Here's how the part is built. I have some questions about the finished solid (model axes, mm). Give positions to 0.01 mm unless a question says otherwise; leave off trailing zeros. Write each loop counter-clockwise with the first axis right and the second up, starting at its lowest first coordinate (ties: lowest second). Pieces come first, ordered by that corner, then holes. Notation, with made-up numbers: M -13.75,-3 L -6.75,-3 A21 cw -6.75,20 Z; hole C 36,79 d10. An arc over 180 degrees is marked long. Use one line per item in the form item = value. Start each with the question number.
Autodesk Inventor part; units mm, degrees
ref_plane "YZ Plane" through (0, 0, 0) normal (1, 0, 0) x (0, 1, 0)
ref_plane "XZ Plane" through (0, 0, 0) normal (0, 1, 0) x (-1, 0, 0)
ref_plane "XY Plane" through (0, 0, 0) normal (0, 0, 1) x (1, 0, 0)
sketch "Sketch1" plane through (0, 0, 0) normal (0, 1, 0) x (-1, 0, 0)
  point P0 (0, 0)
sketch "Sketch4" plane through (0, 0, 0) normal (0, 1, 0) x (-1, 0, 0)
  line L0 (-203.2, 0) -> (-203.2, -254)
  line L1 (-203.2, -254) -> (0, -254)
  line L2 (0, -254) -> (0, 0)
  line L3 (-101.6, 44.45) -> (-50.8, 44.45)
  line L4 (-50.8, 44.45) -> (0, 0)
  line L5 (-101.6, 44.45) -> (-152.4, 44.45)
  line L6 (-152.4, 44.45) -> (-203.2, 0)
  line L7 (-152.4, 44.45) -> (-136.0714, 58.7375)
  line L8 (-50.8, 44.45) -> (-67.1286, 58.7375)
  line L9 (-67.1286, 58.7375) -> (-136.0714, 58.7375)
  line L10 (0, -254) -> (0, -241.3)
  line L11 (-3.175, -241.3) -> (-3.175, -222.25)
  line L12 (-3.175, -222.25) -> (-9.525, -222.25)
  line L13 (-9.525, -222.25) -> (-9.525, -241.3)
  line L14 (-9.525, -241.3) -> (-3.175, -241.3)
  circle A0 centre (-6.35, -215.9) radius 4.7625
  circle A1 centre (-6.35, -215.9) radius 1.9844
  line L15 (-6.35, -209.55) -> (-9.525, -209.55)
  line L16 (-6.35, -209.55) -> (-3.175, -209.55)
  line L17 (-3.175, -209.55) -> (-3.175, -190.5)
  line L18 (-3.175, -190.5) -> (-9.525, -190.5)
  line L19 (-9.525, -190.5) -> (-9.525, -209.55)
  line L20 (-200.025, -241.3) -> (-200.025, -222.25)
  line L21 (-200.025, -222.25) -> (-193.675, -222.25)
  line L22 (-193.675, -222.25) -> (-193.675, -241.3)
  line L23 (-193.675, -241.3) -> (-200.025, -241.3)
  circle A2 centre (-196.85, -215.9) radius 4.7625
  circle A3 centre (-196.85, -215.9) radius 1.9844
  line L24 (-196.85, -209.55) -> (-193.675, -209.55)
  line L25 (-196.85, -209.55) -> (-200.025, -209.55)
  line L26 (-200.025, -209.55) -> (-200.025, -190.5)
  line L27 (-200.025, -190.5) -> (-193.675, -190.5)
  line L28 (-193.675, -190.5) -> (-193.675, -209.55)
  line L29 (-3.175, -63.5) -> (-3.175, -82.55)
  line L30 (-3.175, -82.55) -> (-9.525, -82.55)
  line L31 (-9.525, -82.55) -> (-9.525, -63.5)
  line L32 (-9.525, -63.5) -> (-3.175, -63.5)
  circle A4 centre (-6.35, -88.9) radius 4.7625
  circle A5 centre (-6.35, -88.9) radius 1.9844
  line L33 (-6.35, -95.25) -> (-9.525, -95.25)
  line L34 (-6.35, -95.25) -> (-3.175, -95.25)
  line L35 (-3.175, -95.25) -> (-3.175, -114.3)
  line L36 (-3.175, -114.3) -> (-9.525, -114.3)
  line L37 (-9.525, -114.3) -> (-9.525, -95.25)
  line L38 (-193.675, -63.5) -> (-200.025, -63.5)
  line L39 (-200.025, -63.5) -> (-200.025, -82.55)
  line L40 (-193.675, -82.55) -> (-193.675, -63.5)
  line L41 (-200.025, -82.55) -> (-193.675, -82.55)
  circle A6 centre (-196.85, -88.9) radius 4.7625
  line L42 (-196.85, -95.25) -> (-200.025, -95.25)
  line L43 (-196.85, -95.25) -> (-193.675, -95.25)
  line L44 (-200.025, -95.25) -> (-200.025, -114.3)
  line L45 (-200.025, -114.3) -> (-193.675, -114.3)
  line L46 (-193.675, -114.3) -> (-193.675, -95.25)
  circle A7 centre (-196.85, -88.9) radius 1.9844
  dimension "d18" = 203.2
  dimension "d19" = 254
  dimension "d29" = 19.05
  dimension "d30" = 6.35
  dimension "d32" = 9.525
  dimension "d33" = 3.9688
  dimension "d35" = 3.175
  dimension "d36" = 19.05
extrude "Extrusion2" add sketch "Sketch4" along normal blind 5.5563 contours L6 L5 L3 L4 L2 L1 L0 | L7 L9 L8 L3 L5 | A0 | A2 | A4 | A6
sketch "Sketch5" plane through (0, 5.5563, 0) normal (0, 1, 0) x (1, 0, 0)
  line L0 (67.1286, -58.7375) -> (136.0714, -58.7375)
  line L1 (136.0714, -58.7375) -> (129.7214, -58.7375)
  line L2 (129.7214, -58.7375) -> (129.7214, -52.3875)
  line L3 (129.7214, -52.3875) -> (117.0214, -52.3875)
  line L4 (117.0214, -52.3875) -> (117.0214, -58.7375)
  line L5 (117.0214, -58.7375) -> (104.3214, -58.7375)
  line L6 (0, 0) -> (67.1286, -58.7375)
  line L7 (67.1286, -58.7375) -> (73.4786, -58.7375)
  line L8 (73.4786, -58.7375) -> (73.4786, -52.3875)
  line L9 (73.4786, -52.3875) -> (86.1786, -52.3875)
  line L10 (86.1786, -52.3875) -> (86.1786, -58.7375)
  line L11 (86.1786, -58.7375) -> (101.5964, -58.7375)
  line L12 (101.5964, -52.3875) -> (95.2464, -52.3875)
  line L13 (101.5964, -52.3875) -> (107.9464, -52.3875)
  line L14 (107.9464, -52.3875) -> (107.9464, -58.7375)
  line L15 (95.2464, -52.3875) -> (95.2464, -58.7375)
  line L16 (73.4786, -58.7375) -> (86.1786, -58.7375)
extrude "Extrusion3" cut sketch "Sketch5" against normal blind 25.4
sketch "Sketch6" plane through (0, 5.5563, 0) normal (0, 1, 0) x (1, 0, 0)
  line L0 (73.4786, -52.3875) -> (86.1786, -52.3875)
  line L1 (73.4786, -46.0375) -> (73.4786, -39.6875)
  line L2 (73.4786, -39.6875) -> (73.4786, -46.0375)
  line L3 (129.74, -46.0375) -> (129.74, -39.6875)
  line L4 (129.74, -39.6875) -> (129.74, -46.0375)
  line L5 (86.1786, -46.0375) -> (86.1786, -39.6875)
  line L6 (95.2464, -46.0375) -> (95.2464, -39.6875)
  line L7 (117.0167, -46.0375) -> (117.0167, -39.6875)
  line L8 (107.95, -46.0375) -> (107.95, -39.6875)
  line L9 (73.4786, -39.6875) -> (86.1786, -39.6875)
  line L10 (95.2464, -39.6875) -> (107.95, -39.6875)
  line L11 (117.0167, -39.6875) -> (129.74, -39.6875)
  line L12 (129.74, -46.0375) -> (117.0167, -46.0375)
  line L13 (107.95, -46.0375) -> (95.2464, -46.0375)
  line L14 (86.1786, -46.0375) -> (73.4786, -46.0375)
  point P0 (0, 0)
  point P1 (95.2464, -52.3875)
extrude "Extrusion4" cut sketch "Sketch6" against normal blind 25.4
sketch "Sketch7" plane through (0, 5.5563, 0) normal (0, 1, 0) x (1, 0, 0)
  line L0 (3.175, 63.5) -> (3.175, 82.55)
  line L1 (3.175, 73.025) -> (8.7313, 73.025)
  line L2 (9.525, 82.55) -> (3.175, 82.55)
  line L3 (3.175, 63.5) -> (9.525, 63.5)
  line L4 (9.525, 82.55) -> (8.7313, 82.55)
  line L5 (8.7313, 82.55) -> (8.7313, 63.5)
  line L6 (8.7313, 63.5) -> (9.525, 63.5)
  line L7 (9.525, 63.5) -> (9.525, 82.55)
  line L8 (9.525, 114.3) -> (8.7313, 114.3)
  line L9 (8.7313, 114.3) -> (8.7313, 95.25)
  line L10 (8.7313, 95.25) -> (9.525, 95.25)
  line L11 (9.525, 95.25) -> (9.525, 114.3)
  line L12 (3.175, 209.55) -> (9.525, 209.55)
  line L13 (3.175, 190.5) -> (9.525, 190.5)
  line L14 (9.525, 209.55) -> (8.7313, 209.55)
  line L15 (8.7313, 209.55) -> (8.7313, 190.5)
  line L16 (8.7313, 190.5) -> (9.525, 190.5)
  line L17 (9.525, 190.5) -> (9.525, 209.55)
  line L18 (9.525, 241.3) -> (9.525, 222.25)
  line L19 (9.525, 241.3) -> (9.1281, 241.3)
  line L20 (9.1281, 222.25) -> (9.525, 222.25)
  line L21 (9.525, 222.25) -> (9.525, 241.3)
  line L22 (3.175, 222.25) -> (3.175, 241.3)
  line L23 (9.525, 241.3) -> (8.7313, 241.3)
  line L24 (8.7313, 241.3) -> (8.7313, 222.25)
  line L25 (8.7313, 222.25) -> (9.525, 222.25)
  line L26 (9.525, 222.25) -> (9.525, 241.3)
  line L27 (200.025, 241.3) -> (200.025, 222.25)
  line L28 (200.025, 231.775) -> (194.4688, 231.775)
  line L29 (193.675, 241.3) -> (193.675, 222.25)
  line L30 (193.675, 241.3) -> (194.4688, 241.3)
  line L31 (194.4688, 241.3) -> (194.4688, 222.25)
  line L32 (194.4688, 222.25) -> (193.675, 222.25)
  line L33 (193.675, 222.25) -> (193.675, 241.3)
  line L34 (193.675, 209.55) -> (193.675, 190.5)
  line L35 (200.025, 190.5) -> (193.675, 190.5)
  line L36 (193.675, 209.55) -> (194.4688, 209.55)
  line L37 (194.4688, 209.55) -> (194.4688, 190.5)
  line L38 (194.4688, 190.5) -> (193.675, 190.5)
  line L39 (193.675, 190.5) -> (193.675, 209.55)
  line L40 (193.675, 114.3) -> (194.4688, 114.3)
  line L41 (194.4688, 114.3) -> (194.4688, 95.25)
  line L42 (194.4688, 95.25) -> (193.675, 95.25)
  line L43 (193.675, 95.25) -> (193.675, 114.3)
  line L44 (193.675, 82.55) -> (193.675, 63.5)
  line L45 (193.675, 82.55) -> (194.4688, 82.55)
  line L46 (194.4688, 82.55) -> (194.4688, 63.5)
  line L47 (194.4688, 63.5) -> (193.675, 63.5)
  line L48 (193.675, 63.5) -> (193.675, 82.55)
  line L49 (86.1786, -52.3875) -> (86.1786, -58.7375)
  line L50 (73.4786, -52.3875) -> (73.4786, -58.7375)
  line L51 (86.1786, -52.3875) -> (73.4786, -52.3875)
  line L52 (73.4786, -52.3875) -> (73.4786, -53.1813)
  line L53 (73.4786, -53.1813) -> (86.1786, -53.1813)
  line L54 (86.1786, -53.1813) -> (86.1786, -52.3875)
  line L55 (95.2464, -58.7375) -> (95.2464, -52.3875)
  line L56 (107.9464, -52.3875) -> (107.9464, -58.7375)
  line L57 (95.2464, -52.3875) -> (107.9464, -52.3875)
  line L58 (107.9464, -52.3875) -> (107.9464, -53.1813)
  line L59 (107.9464, -53.1813) -> (95.2464, -53.1813)
  line L60 (95.2464, -53.1813) -> (95.2464, -52.3875)
  line L61 (117.0214, -52.3875) -> (130.175, -52.3875)
  line L62 (130.175, -52.3875) -> (130.175, -53.1813)
  line L63 (130.175, -53.1813) -> (117.0214, -53.1813)
  line L64 (117.0214, -53.1813) -> (117.0214, -52.3875)
  line L65 (86.1786, -46.0375) -> (86.1786, -39.6875)
  line L66 (73.4786, -39.6875) -> (86.1786, -39.6875)
  line L67 (86.1786, -39.6875) -> (86.1786, -40.4853)
  line L68 (86.1786, -40.4853) -> (73.4786, -40.4853)
  line L69 (73.4786, -40.4853) -> (73.4786, -39.6875)
  line L70 (95.2464, -39.6875) -> (107.9464, -39.6875)
  line L71 (107.9464, -39.6875) -> (107.9464, -40.4853)
  line L72 (107.9464, -40.4853) -> (95.2464, -40.4853)
  line L73 (95.2464, -40.4853) -> (95.2464, -39.6875)
  line L74 (117.0214, -39.6875) -> (129.74, -39.6875)
  line L75 (129.74, -39.6875) -> (129.74, -40.4853)
  line L76 (129.74, -40.4853) -> (117.0214, -40.4853)
  line L77 (117.0214, -40.4853) -> (117.0214, -39.6875)
  point P0 (0, 0)
  dimension "d65" = 5.5563
  dimension "d67" = 5.5563
extrude "Extrusion5" add sketch "Sketch7" against normal blind 5.5563 contours L5 L2 L7 L3 | L11 L10 L9 L8 | L12 L17 L13 L15 | L18 L20 L25 L24 L23 L19 | L30 L31 L32 L29 | L36 L37 L35 L34 | L40 L41 L42 L43 | L45 L46 L47 L44 | L49 L53 L50 L51 | L55 L57 L56 L59 | L61 L62 L63 L64 | L68 L69 L66 L65 | L70 L71 L72 L73 | L74 L75 L76 L77
properties part number "base"
1) Suppose I cut it at C-C, the plane y = 3.4. State how many separate pieces and enclosed holes the cut face has, and give its area (3 significant figures).
2) Will these pins go through, and if not, where does the flat tip stop? P1, Ø3, axis at y = 2, z = 56.5, coming from the +X side; P2, Ø3, axis at x = 76.5, y = 4.5, coming from the +Z side; P3, Ø3, axis at y = 1.5, z = 43, coming from the +X side; P4, Ø2.5, axis at x = 196.85, z = -215.9, coming from the +Y side.
3) Suppose I cut it at A-A, the plane z = -70.5. List the corners of the cut face in (x, y) for me (3 decimals).
4) Suppose I cut it at B-B, the plane x = 122.5. List the corners of the cut face in (y, z) for me, and give its area (3 significant figures).
5) Suppose I cut it at D-D, the plane x = 157. List the corners of the cut face in (y, z) for me (3 decimals).
6) Please list where these lines run through material, in increasing order: line 1 (X direction, y = 2.3, z = -215.9); line 2 (X direction, y = 1.2, z = -236.5) (3 decimals); line 3 (Z direction, x = 138, y = 5.1).
Checks:
q1.separate_pieces = 1
q1.enclosed_holes = 15
q1.area = 58,300 mm^2
q2.P1 = 140.34
q2.P2 = 53.18
q2.P3 = 155.77
q2.P4 = through
q3.outline = M 0,0 L 3.175,0 L 3.175,5.556 L 0,5.556 Z; M 8.731,0 L 194.469,0 L 194.469,5.556 L 8.731,5.556 Z; M 200.025,0 L 203.2,0 L 203.2,5.556 L 200.025,5.556 Z
q4.outline = M 0,-254 L 5.56,-254 L 5.56,40.49 L 0,40.49 Z; M 0,46.04 L 5.56,46.04 L 5.56,53.18 L 0,53.18 Z
q4.area = 1,680 mm^2
q5.outline = M 0,-254 L 5.556,-254 L 5.556,40.425 L 0,40.425 Z
q6.line_1 = 0 to 4.37, 8.33 to 194.87, 198.83 to 203.2
q6.line_2 = 0 to 3.175, 8.731 to 194.469, 200.025 to 203.2
q6.line_3 = -254 to 57.05
